Part model, mm, in its own coordinate system. A direction names the side the tool comes from. Round coordinates to 2 decimals unless told otherwise and drop trailing zeros. Loops run counter-clockwise (first coordinate to the right, second up) from the corner with the lowest first, then second, coordinate; pieces in that order, holes last.
(1) Mould opens along Z. For faces 1 (the face through (-1, 2, 0)), 2 (the face through (1.14, 2.41, -2.17)), 3 (the face through (-1.14, -2.41, -2.17)), 4 (the face through (-2.88, -2.64, -0.28)) say: +Z half, -Z half, draft (parallel to the pull), parting line (faces both ways), or undercut.
(2) Flat gauge pin, fed straight in: pin 1 (1 mm diameter, centred on y = 1.5, z = -2.5, fed in from +X). Where does the tip first touch, or does it go through?
(3) Tool access for faces 5 (the face through (-1.905, -0.084, -4.198)), 6 (the face through (-0.014, 2.667, -2.168)): list every direction of +Z, -Z, +X, -X, +Y, -Y with a clear straight run to the whole face (end or side of a thin tool).
(4) Cut at D-D on y = 3.5. List the corners of the cut face in (x, z), then the cut area to 3 significant figures.
(5) Cut at B-B on y = 0. List the corners of the cut face in (x, z).
(6) Cut at A-A on x = 0. List the corners of the cut face in (y, z).
(7) Probe probe 1 along Z at (x, y) = (-3.5, 1); probe 2 along Y at (x, z) = (-2.75, -3.75); probe 3 along Y at (x, z) = (1.75, -1.25). List the from-to ranges inside material, lowest first.
from build123d import *

# Parameters (mm, degrees)
CUT_EXTRUDE1_START = 3.229191933
CUT_EXTRUDE1_DEPTH = 3.229191933


with BuildPart() as part:
    # Sketch1 → Revolve2 (revolve)
    with BuildSketch(Plane(origin=(0, 0, 0), x_dir=(0, 0, -1), z_dir=(1, 0, 0)), mode=Mode.PRIVATE) as revolve2_sk:
        Polygon((4.77917475, 3.907122765), (3.805254495, 3.907122765), (3.805254495, 3.407122765), (0.576062562, 3.407122765), (0.576062562, 3.907122765), (0, 3.907122765), (0, 1.907122765), (4.77917475, 1.907122765), (8.27917475, 1.907122765), (8.27917475, 3.753666669), (8.27917475, 3.907122765), align=None)
    revolve(revolve2_sk.sketch.rotate(Axis((0, 0, 0), (0, 0, -1)), 90), axis=Axis((0, 0, 0), (0, 0, -1)))

    # Sketch3 → Cut-Extrude1 (cut)
    with BuildSketch(Plane.XY.offset(-3.805254495).offset(CUT_EXTRUDE1_START)):
        with BuildLine():
            ThreePointArc((-2.301258727, 2.512507474), (-2.663795842, 2.124306298), (-2.961591907, 1.684475857))
            ThreePointArc((-2.961591907, 1.684475857), (-2.085240545, 1.662923844), (-2.301258727, 2.512507474))
        make_face()
        with BuildLine():
            ThreePointArc((-0.529546095, 3.365719309), (0, 2.667122765), (0.529546095, 3.365719309))
            ThreePointArc((0.529546095, 3.365719309), (0, 3.407122765), (-0.529546095, 3.365719309))
        make_face()
        with BuildLine():
            ThreePointArc((0.983226333, 3.262169756), (1.157221198, 2.402994578), (1.937435425, 2.802646876))
            ThreePointArc((1.937435425, 2.802646876), (1.478295165, 3.06971154), (0.983226333, 3.262169756))
        make_face()
        with BuildLine():
            ThreePointArc((2.301258727, 2.512507474), (2.085240545, 1.662923844), (2.961591907, 1.684475857))
            ThreePointArc((2.961591907, 1.684475857), (2.663795842, 2.124306298), (2.301258727, 2.512507474))
        make_face()
        with BuildLine():
            ThreePointArc((3.163498608, 1.265212273), (2.600252429, 0.593490649), (3.399168791, 0.232673735))
            ThreePointArc((3.399168791, 0.232673735), (3.321699084, 0.75815614), (3.163498608, 1.265212273))
        make_face()
        with BuildLine():
            ThreePointArc((3.399168791, -0.232673735), (2.600252429, -0.593490649), (3.163498608, -1.265212273))
            ThreePointArc((3.163498608, -1.265212273), (3.321699084, -0.75815614), (3.399168791, -0.232673735))
        make_face()
        with BuildLine():
            ThreePointArc((2.961591907, -1.684475857), (2.085240545, -1.662923844), (2.301258727, -2.512507474))
            ThreePointArc((2.301258727, -2.512507474), (2.663795842, -2.124306298), (2.961591907, -1.684475857))
        make_face()
        with BuildLine():
            ThreePointArc((1.937435425, -2.802646876), (1.157221198, -2.402994578), (0.983226333, -3.262169756))
            ThreePointArc((0.983226333, -3.262169756), (1.478295165, -3.06971154), (1.937435425, -2.802646876))
        make_face()
        with BuildLine():
            ThreePointArc((0.529546095, -3.365719309), (0, -2.667122765), (-0.529546095, -3.365719309))
            ThreePointArc((-0.529546095, -3.365719309), (0, -3.407122765), (0.529546095, -3.365719309))
        make_face()
        with BuildLine():
            ThreePointArc((-0.983226333, -3.262169756), (-1.157221198, -2.402994578), (-1.937435425, -2.802646876))
            ThreePointArc((-1.937435425, -2.802646876), (-1.478295165, -3.06971154), (-0.983226333, -3.262169756))
        make_face()
        with BuildLine():
            ThreePointArc((-2.301258727, -2.512507474), (-2.085240545, -1.662923844), (-2.961591907, -1.684475857))
            ThreePointArc((-2.961591907, -1.684475857), (-2.663795842, -2.124306298), (-2.301258727, -2.512507474))
        make_face()
        with BuildLine():
            ThreePointArc((-3.163498608, -1.265212273), (-2.600252429, -0.593490649), (-3.399168791, -0.232673735))
            ThreePointArc((-3.399168791, -0.232673735), (-3.321699084, -0.75815614), (-3.163498608, -1.265212273))
        make_face()
        with BuildLine():
            ThreePointArc((-3.399168791, 0.232673735), (-2.600252429, 0.593490649), (-3.163498608, 1.265212273))
            ThreePointArc((-3.163498608, 1.265212273), (-3.321699084, 0.75815614), (-3.399168791, 0.232673735))
        make_face()
        with BuildLine():
            ThreePointArc((-1.937435425, 2.802646876), (-1.157221198, 2.402994578), (-0.983226333, 3.262169756))
            ThreePointArc((-0.983226333, 3.262169756), (-1.478295165, 3.06971154), (-1.937435425, 2.802646876))
        make_face()
    extrude(amount=-CUT_EXTRUDE1_DEPTH, mode=Mode.SUBTRACT)


solid = part.part
Final values:
1. face 1: +Z half
1. face 2: undercut
1. face 3: undercut
1. face 4: draft
2. pin 1: stops at x = 3.16
3. face 5: +Z, -Z
3. face 6: none
4. outline: (-1.74, -8.28) - (1.74, -8.28) - (1.74, -3.81) - (-1.74, -3.81) - close; (-1.74, -0.58) - (1.74, -0.58) - (1.74, 0) - (-1.74, 0) - close
4. area: 17.5 mm2
5. outline: (-3.91, -8.28) - (-1.91, -8.28) - (-1.91, 0) - (-3.91, 0) - (-3.91, -0.58) - (-3.41, -0.58) - (-3.41, -3.81) - (-3.91, -3.81) - close; (1.91, -8.28) - (3.91, -8.28) - (3.91, -3.81) - (3.41, -3.81) - (3.41, -0.58) - (3.91, -0.58) - (3.91, 0) - (1.91, 0) - close
6. outline: (-3.91, -8.28) - (-1.91, -8.28) - (-1.91, 0) - (-3.91, 0) - (-3.91, -0.58) - (-2.67, -0.58) - (-2.67, -3.81) - (-3.91, -3.81) - close; (1.91, -8.28) - (3.91, -8.28) - (3.91, -3.81) - (2.67, -3.81) - (2.67, -0.58) - (3.91, -0.58) - (3.91, 0) - (1.91, 0) - close
7. probe 1: z = -8.28 to -3.81, -0.58 to 0
7. probe 2: y = -1.51 to -1.11, -0.32 to 0.32, 1.11 to 1.51
7. probe 3: y = -2.48 to -0.76, 0.76 to 2.48
